For this review, take the finished solid that the model builds, in its own axes (mm). A direction names the side the tool comes from. Coordinates: 2 decimals unless noted, no trailing zeros. Loops run counter-clockwise (first coordinate to the right, second up) from the corner with the lowest first, then second, coordinate; pieces in that order, holes last. Notation, with made-up numbers: (81.5, 89.25) -> (140.5, 89.25) arc R31 ccw to (140.5, 121.25) -> close; hole circle Ø7 at (80.5, -24). An arc over 180 degrees is marked (long way). Use a Markdown table: item, result.
from build123d import *

# Parameters (mm, degrees)
SHANK_PROFILE_R = 3
SHANK_DEPTH     = 25
HEAD_START      = 25
HEAD_DEPTH      = 4


with BuildPart() as part:
    # Shank Profile → Shank (new body)
    with BuildSketch(Plane(origin=(0, 0, 0), x_dir=(1, 0, 0), z_dir=(0, 1, 0))):
        with Locations(Location((0, 0, 0), (0, 0, 270))):
            Circle(SHANK_PROFILE_R)
    extrude(amount=SHANK_DEPTH)

    # Head Profile → Head (add)
    with BuildSketch(Plane(origin=(0, 0, 0), x_dir=(1, 0, 0), z_dir=(0, 1, 0)).offset(HEAD_START)):
        Polygon((5.773502692, 0), (2.886751346, -5), (-2.886751346, -5), (-5.773502692, 0), (-2.886751346, 5), (2.886751346, 5), align=None)
    extrude(amount=HEAD_DEPTH)


solid = part.part
(1) Take a section at A-A on x = 0. Write out the cut boundary in (y, z).
Found:
| item | result |
|---|---|
| outline | (0, -3) -> (25, -3) -> (25, -5) -> (29, -5) -> (29, 5) -> (25, 5) -> (25, 3) -> (0, 3) -> close |
(2) For pin 1 Ø3 at (x, y) = (1, 20.5) entering from +Z; pin 2 Ø6 at (y, z) = (6.5, -3.5) entering from +X; pin 3 Ø3 at (x, y) = (1, 22.5) entering from -Z, all flat-tipped, find the tip position at first contact; note any pin that passes through.
Found:
| item | result |
|---|---|
| pin 1 | stops at z = 3 |
| pin 2 | stops at x = 2.96 |
| pin 3 | stops at z = -3 |
(3) Take a section at B-B on z = 2.5. Write out the cut boundary in (x, y).
Found:
| item | result |
|---|---|
| outline | (-4.33, 25) -> (-1.66, 25) -> (-1.66, 0) -> (1.66, 0) -> (1.66, 25) -> (4.33, 25) -> (4.33, 29) -> (-4.33, 29) -> close |
(4) For faces 1 (the face through (0.9, 12.32, 2.86)), 2 (the face through (-4.31, 26.972, 2.535)), list the 3-axis set-ups (+Z, -Z, +X, -X, +Y, -Y) from which the entire face can be reached by the end or side of a thin tool; tool diameter is ignored.
Found:
| item | result |
|---|---|
| face 1 | -Y |
| face 2 | +Z, -X, +Y, -Y |
(5) Take a section at D-D on x = 5. Write out the cut boundary in (y, z), plus the area to 3 significant figures.
Found:
| item | result |
|---|---|
| outline | (25, -1.34) -> (29, -1.34) -> (29, 1.34) -> (25, 1.34) -> close |
| area | 10.7 mm^2 |
(6) Take a section at C-C on y = 20. Write out the cut boundary in (x, z), plus the area to 3 significant figures.
Found:
| item | result |
|---|---|
| outline | circle Ø6 at (0, 0) |
| area | 28.3 mm^2 |
(7) For line 1 along Y through (x, z) = (3, 4.25); line 2 along X through (y, z) = (17.5, 0); line 3 along X through (y, z) = (25.75, 4.25), list the stretches that pass through material, from the lowest coordinate up.
Found:
| item | result |
|---|---|
| line 1 | y = 25 to 29 |
| line 2 | x = -3 to 3 |
| line 3 | x = -3.32 to 3.32 |
